The model under review builds one solid part; all positions refer to its coordinate system, in mm. Face numbers are marked on the shaded views. A direction names the side the tool comes from. Give positions to 0.01 mm unless a question says otherwise; leave off trailing zeros. Loops run counter-clockwise (first coordinate to the right, second up) from the corner with the lowest first, then second, coordinate; pieces in that order, holes last. Notation, with made-up numbers: M 60,54.5 L 119,54.5 A15 ccw 119,81.5 Z; hole C 15,-39.5 d8. An arc over 180 degrees is marked long. Return JSON: item names as keys, results as strings. Group by question number.
```python
from build123d import *

# Parameters (mm, degrees)
F1_DEPTH = 25.4
F3_DEPTH = 2.54
F4_SIZE  = 5.08
F5_DEPTH = 25.4


with BuildPart() as f1:
    # F0 (on Right) → F1 (new body, symmetric)
    with BuildSketch(Plane.YZ):
        Polygon((-14.806319427, 59.3731885201), (-55.446319427, 59.3731885201), (-55.446319427, -108.2668114799), (-4.646319427, -108.2668114799), (-4.646319427, -57.4668114799), (6.8900182168, -40.7391304162), (6.8900182168, -0.0991304162), (-33.7499817832, -0.0991304162), (-39.8801730554, 40.0758662231), (-14.806319427, 44.1331885201), align=None)
    extrude(amount=F1_DEPTH, both=True)

    # F2 (on face) → F3 (join, symmetric)
    with BuildSketch(Plane.XY.offset(-0.0991304162)):
        Polygon((-37.2138172336, -33.7499817832), (38.9861827664, -33.7499817832), (38.9861827664, -3.4425283198), (28.0170366168, 6.8900182168), (-37.2138172336, 6.8900182168), align=None)
    extrude(amount=F3_DEPTH, both=True)

    # F4
    f4_edges = [f1.edges().sort_by_distance(p)[0] for p in [
        (38.986183, -33.749982, -0.09913),
    ]]
    chamfer(f4_edges, length=F4_SIZE)

    # F0 (on Right) → F5 (join)
    with BuildSketch(Plane.YZ):
        Polygon((-14.806319427, 59.3731885201), (-55.446319427, 59.3731885201), (-55.446319427, -108.2668114799), (-4.646319427, -108.2668114799), (-4.646319427, -57.4668114799), (6.8900182168, -40.7391304162), (6.8900182168, -0.0991304162), (-33.7499817832, -0.0991304162), (-39.8801730554, 40.0758662231), (-14.806319427, 44.1331885201), align=None)
    extrude(amount=F5_DEPTH)


solid = f1.part
```
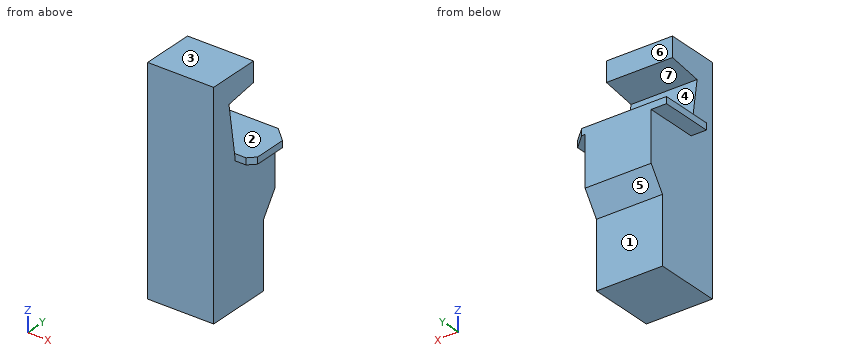
(1) For the marked faces 1, 2 and 3, list the 3-axis set-ups (+Z, -Z, +X, -X, +Y, -Y) from which the entire face can be reached by the end or side of a thin tool; tool diameter is ignored.
(2) For probe 1 along X at (y, z) = (-31, -70); probe 2 along Z at (x, y) = (-30, -24); probe 3 along Z at (x, y) = (-20, -8.5), list the stretches that pass through material, from the lowest coordinate up.
(3) Add section B-B (x = -3). Write out the cut boundary in (y, z), and give its area (3 significant figures).
(4) Add section D-D (y = 1). Write out the cut boundary in (x, z).
(5) For pin 1 (12 mm diameter, centred on x = -23.5, y = -2.5, fed in from +Z); pin 2 (4 mm diameter, centred on y = -5.5, z = -90.5, fed in from +X); pin 3 (12 mm diameter, centred on x = 3, z = 52.5, fed in from +Y), all flat-tipped, find the tip position at first contact; note any pin that passes through.
(6) Add section A-A (y = -7.5). Write out the cut boundary in (x, z).
(7) Mouldability with a two-part tool opening along Z and no side actions: class the marked faces 4, 5, 6 and 7 as released by +Z, released by -Z, zero draft, split by the parting line, or undercut.
(8) Add section C-C (z = -70). Write out the cut boundary in (x, y).
Verdict:
{
 "1": {"face 1": "-Z, +X, -X, +Y", "face 2": "+X, -X, +Y", "face 3": "+Z, +X, -X, +Y, -Y"},
 "2": {"probe 1": "x = -25.4 to 25.4", "probe 2": "z = -2.64 to 2.44", "probe 3": "z = -108.27 to 2.44"},
 "3": {"outline": "M -55.45,-108.27 L -4.65,-108.27 L -4.65,-57.47 L 6.89,-40.74 L 6.89,2.44 L -33.75,2.44 L -33.75,-0.1 L -39.88,40.08 L -14.81,44.13 L -14.81,59.37 L -55.45,59.37 Z", "area": "7,650 mm²"},
 "4": {"outline": "M -37.21,-2.64 L -25.4,-2.64 L -25.4,-49.28 L 25.4,-49.28 L 25.4,-2.64 L 34.27,-2.64 L 34.27,2.44 L -37.21,2.44 Z"},
 "5": {"pin 1": "stops at z = 2.44", "pin 2": "stops at x = 25.4", "pin 3": "stops at y = -14.81"},
 "6": {"outline": "M -37.21,-2.64 L -25.4,-2.64 L -25.4,-108.27 L 25.4,-108.27 L 25.4,-2.64 L 38.99,-2.64 L 38.99,2.44 L -37.21,2.44 Z"},
 "7": {"face 4": "undercut", "face 5": "released by -Z", "face 6": "zero draft", "face 7": "undercut"},
 "8": {"outline": "M -25.4,-55.45 L 25.4,-55.45 L 25.4,-4.65 L -25.4,-4.65 Z"}
}
